from build123d import *

# Parameters (mm, degrees)
SKETCH1_W      = 18.288
SKETCH1_H      = 6.858
EXTRUDE1_DEPTH = 3.048
SKETCH2_W      = 0.762
SKETCH2_H      = 0.762
EXTRUDE2_DEPTH = 7.62


with BuildPart() as part:
    # Sketch1 → Extrude1 (new body)
    with BuildSketch(Plane(origin=(0, 0, 0), x_dir=(1, 0, 0), z_dir=(0, 1, 0))):
        with Locations((9.144, 3.429)):
            Rectangle(SKETCH1_W, SKETCH1_H)
    extrude(amount=EXTRUDE1_DEPTH)

    # Sketch2 → Extrude2 (add)
    with BuildSketch(Plane(origin=(0, 3.048, 0), x_dir=(1, 0, 0), z_dir=(0, 1, 0))):
        with Locations((3.429, 5.715)):
            Rectangle(SKETCH2_W, SKETCH2_H)
        with Locations((1.143, 5.715)):
            Rectangle(SKETCH2_W, SKETCH2_H)
        with Locations((5.715, 5.715)):
            Rectangle(SKETCH2_W, SKETCH2_H)
        with Locations((8.001, 5.715)):
            Rectangle(SKETCH2_W, SKETCH2_H)
        with Locations((10.287, 5.715)):
            Rectangle(SKETCH2_W, SKETCH2_H)
        with Locations((12.573, 5.715)):
            Rectangle(SKETCH2_W, SKETCH2_H)
        with Locations((14.859, 5.715)):
            Rectangle(SKETCH2_W, SKETCH2_H)
        with Locations((17.145, 5.715)):
            Rectangle(SKETCH2_W, SKETCH2_H)
        with Locations((1.143, 3.429)):
            Rectangle(SKETCH2_W, SKETCH2_H)
        with Locations((3.429, 3.429)):
            Rectangle(SKETCH2_W, SKETCH2_H)
        with Locations((5.715, 3.429)):
            Rectangle(SKETCH2_W, SKETCH2_H)
        with Locations((8.001, 3.429)):
            Rectangle(SKETCH2_W, SKETCH2_H)
        with Locations((10.287, 3.429)):
            Rectangle(SKETCH2_W, SKETCH2_H)
        with Locations((12.573, 3.429)):
            Rectangle(SKETCH2_W, SKETCH2_H)
        with Locations((14.859, 3.429)):
            Rectangle(SKETCH2_W, SKETCH2_H)
        with Locations((17.145, 3.429)):
            Rectangle(SKETCH2_W, SKETCH2_H)
        with Locations((1.143, 1.143)):
            Rectangle(SKETCH2_W, SKETCH2_H)
        with Locations((3.429, 1.143)):
            Rectangle(SKETCH2_W, SKETCH2_H)
        with Locations((5.715, 1.143)):
            Rectangle(SKETCH2_W, SKETCH2_H)
        with Locations((8.001, 1.143)):
            Rectangle(SKETCH2_W, SKETCH2_H)
        with Locations((10.287, 1.143)):
            Rectangle(SKETCH2_W, SKETCH2_H)
        with Locations((12.573, 1.143)):
            Rectangle(SKETCH2_W, SKETCH2_H)
        with Locations((14.859, 1.143)):
            Rectangle(SKETCH2_W, SKETCH2_H)
        with Locations((17.145, 1.143)):
            Rectangle(SKETCH2_W, SKETCH2_H)
    extrude(amount=EXTRUDE2_DEPTH)


solid = part.part
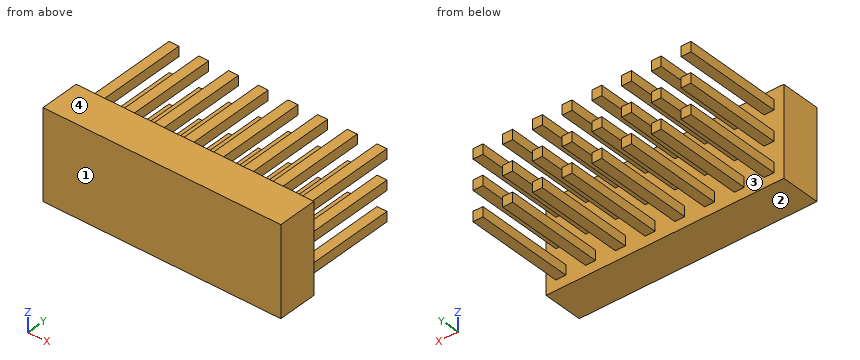
Could you check a few things on this model? Use its own coordinates, in mm. Face numbers are marked on the shaded views. Coordinates: 2 decimals unless noted, no trailing zeros. Loops run counter-clockwise (first coordinate to the right, second up) from the corner with the lowest first, then second, coordinate; pieces in that order, holes last.
1. For P1, Ø0.8, axis at y = 6.5, z = -5.5, coming from the -X side; P2, Ø0.8, axis at x = 10.5, y = 8, coming from the +Z side; P3, Ø2, axis at x = 13.5, y = 5, coming from the -Z side, each with a flat end and sliding along its axis, tell me the tip position at first contact or that it passes through.
2. We'd pull the mould along Z, two halves only. Please class the marked faces 1, 2, 3 and 4: released by +Z, released by -Z, zero draft, split by the parting line, or undercut.
3. Imagine slicing it at C-C (z = -6.5). Please give me the cut outline in (x, y), and give its area (3 significant figures).
4. I need wall thicknesses on L1, parallel to Z at x = 12.25, y = 4; L2, parallel to Y at x = 2, z = -3.75. Which ranges of each line are inside material? Lowest first, please.
5. Imagine slicing it at B-B (y = 3.25). Give the number of separate pieces and of enclosed holes in the cut face, and give its area (3 significant figures).
6. Imagine slicing it at A-A (x = 15). Please give me the cut outline in (y, z).
Computed values:
1. P1: stops at x = 0.76
1. P2: stops at z = -0.76
1. P3: stops at z = -6.1
2. face 1: zero draft
2. face 2: released by -Z
2. face 3: undercut
2. face 4: released by +Z
3. outline: (0, 0) - (18.29, 0) - (18.29, 3.05) - (0, 3.05) - close
3. area: 55.7 mm2
4. L1: z = -6.1 to -5.33, -3.81 to -3.05, -1.52 to -0.76
4. L2: y = 0 to 3.05
5. separate pieces: 24
5. enclosed holes: 0
5. area: 13.9 mm2
6. outline: (0, -6.86) - (3.05, -6.86) - (3.05, -6.1) - (10.67, -6.1) - (10.67, -5.33) - (3.05, -5.33) - (3.05, -3.81) - (10.67, -3.81) - (10.67, -3.05) - (3.05, -3.05) - (3.05, -1.52) - (10.67, -1.52) - (10.67, -0.76) - (3.05, -0.76) - (3.05, 0) - (0, 0) - close
